The model under review builds one solid part; all positions refer to its coordinate system, in mm. A direction names the side the tool comes from. Give positions to 0.01 mm unless a question says otherwise; leave off trailing zeros. Order: outer loops, then holes, each group sorted by start corner. A loop starts at its lowest first (then second) coordinate and runs counter-clockwise, first axis right, second up. Notation, with made-up numbers: (35.5, 81) - (88.5, 81) arc R6 cw to (88.5, 86) - close; hole circle Ø11 at (46, 62). An arc over 180 degrees is marked (long way). Use CSV: the item, a comma, the result in double quotes. Start each with the question number.
1. To check wall thickness, follow line 1 (Y direction, x = 4.85, z = -15); line 2 (Y direction, x = 3.9, z = -29); line 3 (Z direction, x = 5.7, y = 17). State the ranges of each line that lie inside material, in increasing order. Write a range as [from, to].
2. Machinability: for faces 5 (the flat face through (3, 53, -20)), 6 (the flat face through (6, 28, -20)), 7 (the flat face through (3, 50, -5)), which of the approach directions +Z, -Z, +X, -X, +Y, -Y give a long, thin tool a straight path to every point of the face, cutting with its end or side? Answer none if there is none.
3. Take a section at B-B, the plane y = 19.5. State the section outline as (x, z) points.
4. Take a section at D-D, the plane x = 2.1. State the section outline as (y, z) points, then the cut area to 3 significant figures.
5. Take a section at C-C, the plane y = 52.5. State the section outline as (x, z) points, then the cut area to 3 significant figures.
6. Take a section at A-A, the plane z = -29. State the section outline as (x, y) points.
7. Draft analysis for pull direction Z (two halves, no side actions). For faces 1 (the cylindrical face through (3, 17.7, -12.6)), 2 (the flat face through (3, 56, -15)), 3 (the flat face through (3, 25, 0)), 4 (the flat face through (3, 28, -40)), state which applies: released by +Z, released by -Z, zero draft, split by the parting line, or undercut.
Autodesk Inventor part; units mm, degrees
ref_plane "YZ Plane" through (0, 0, 0) normal (1, 0, 0) x (0, 1, 0)
ref_plane "XZ Plane" through (0, 0, 0) normal (0, 1, 0) x (-1, 0, 0)
ref_plane "XY Plane" through (0, 0, 0) normal (0, 0, 1) x (1, 0, 0)
sketch "Sketch1" plane through (0, 0, 0) normal (1, 0, 0) x (0, 1, 0)
  line L0 (0, 0) -> (56, 0)
  line L1 (56, 0) -> (56, -40)
  line L2 (56, -40) -> (0, -40)
  line L3 (0, -40) -> (0, 0)
  dimension "d0" = 56
  dimension "d1" = 40
extrude "Extrusion1" add sketch "Sketch1" along normal blind 6
sketch "Sketch2" plane through (6, 0, 0) normal (1, 0, 0) x (0, 0, -1)
  line L0 (40, 56) -> (0, 56)
  line L1 (40, 56) -> (30, 56)
  line L2 (30, 56) -> (20, 56)
  line L3 (20, 56) -> (20, 50)
  line L4 (20, 50) -> (30, 50)
  line L5 (30, 50) -> (30, 56)
  point P0 (0, 0)
  dimension "d4" = 10
  dimension "d5" = 10
  dimension "d6" = 6
extrude "Extrusion2" cut sketch "Sketch2" against normal blind 6
pattern_linear "Rectangular Pattern1" count 2 spacing 20 along (0, 0, 1) of "Extrusion2"
sketch "Sketch3" plane through (6, 0, 0) normal (1, 0, 0) x (0, 0, -1)
  line L0 (30, 50) -> (30, 56)
  circle A0 centre (15, 41.5) radius 3
  circle A1 centre (29, 41.5) radius 3
  circle A2 centre (15, 19.5) radius 3
  circle A3 centre (29, 19.5) radius 3
  point P0 (0, 0)
  dimension "d14" = 6
  dimension "d16" = 6
  dimension "d18" = 6
  dimension "d19" = 6
extrude "Extrusion3" cut sketch "Sketch3" against normal blind 6
properties part number "e_arm holder 2"
Determined:
1,line 1,"y = [0, 16.5], [22.5, 38.5], [44.5, 56]"
1,line 2,"y = [0, 16.5], [22.5, 38.5], [44.5, 50]"
1,line 3,"z = [-40, -30.66], [-27.34, -16.66], [-13.34, 0]"
2,face 5,"+X, -X, +Y"
2,face 6,"+Z, -Z, +X, +Y, -Y"
2,face 7,"+Z, +X, -X, +Y"
3,outline,"(0, -40) - (6, -40) - (6, -32) - (0, -32) - close; (0, -26) - (6, -26) - (6, -18) - (0, -18) - close; (0, -12) - (6, -12) - (6, 0) - (0, 0) - close"
4,outline,"(0, -40) - (56, -40) - (56, -30) - (50, -30) - (50, -20) - (56, -20) - (56, -10) - (50, -10) - (50, 0) - (0, 0) - close; hole circle Ø6 at (19.5, -29); hole circle Ø6 at (19.5, -15); hole circle Ø6 at (41.5, -29); hole circle Ø6 at (41.5, -15)"
4,area,"2,010 mm²"
5,outline,"(0, -40) - (6, -40) - (6, -30) - (0, -30) - close; (0, -20) - (6, -20) - (6, -10) - (0, -10) - close"
5,area,"120 mm²"
6,outline,"(0, 0) - (6, 0) - (6, 16.5) - (0, 16.5) - close; (0, 22.5) - (6, 22.5) - (6, 38.5) - (0, 38.5) - close; (0, 44.5) - (6, 44.5) - (6, 50) - (0, 50) - close"
7,face 1,"undercut"
7,face 2,"zero draft"
7,face 3,"released by +Z"
7,face 4,"released by -Z"
